Autodesk Inventor part; units mm, degrees
ref_plane "YZ Plane" through (0, 0, 0) normal (1, 0, 0) x (0, 1, 0)
ref_plane "XZ Plane" through (0, 0, 0) normal (0, 1, 0) x (-1, 0, 0)
ref_plane "XY Plane" through (0, 0, 0) normal (0, 0, 1) x (1, 0, 0)
sketch "Sketch9" plane through (0, 0, 0) normal (0, 1, 0) x (-1, 0, 0)
  line L0 (30, 30) -> (-30, 30)
  line L1 (-30, 30) -> (-30, -30)
  line L2 (-30, -30) -> (30, -30)
  line L3 (30, -30) -> (30, 30)
  line L4 (30, 30) -> (-30, -30) construction
  line L5 (-30, 30) -> (30, -30) construction
  line L6 (-28, 28) -> (28, 28)
  line L7 (28, 28) -> (28, -28)
  line L8 (28, -28) -> (-28, -28)
  line L9 (-28, -28) -> (-28, 28)
  point P0 (0, 0)
  dimension "d172" = 60
  dimension "d173" = 60
  dimension "d174" = 2
extrude "Extrusion3" add sketch "Sketch9" against normal blind 330
sketch "Sketch10" plane through (0, 0, 0) normal (1, 0, 0) x (0, 1, 0)
  line L0 (0, 30) -> (0, -30) construction
  line L1 (0, 30) -> (-330, 30) construction
  line L2 (-330, -30) -> (-330, 30) construction
  line L3 (0, -30) -> (-330, -30) construction
  line L4 (0, 0) -> (40, 0)
  line L5 (-85.25, -15.25) -> (-85.25, 15.25)
  line L6 (-85.25, 15.25) -> (-54.75, 15.25)
  line L7 (-54.75, 15.25) -> (-54.75, -15.25)
  line L8 (-54.75, -15.25) -> (-85.25, 15.25) construction
  line L9 (-85.25, -15.25) -> (-54.75, 15.25) construction
  circle A0 centre (-93, 23) radius 2.5
  circle A1 centre (-47, 23) radius 2.5
  line L10 (-85.25, -15.25) -> (-93, -23) construction
  circle A2 centre (-47, -23) radius 2.5
  circle A3 centre (-93, -23) radius 2.5
  circle A4 centre (-70, 0) radius 32.5269 construction
  line L11 (-54.75, -15.25) -> (-85.25, -15.25)
  line L12 (-44.5, -25.5) -> (-95.5, -25.5) construction
  line L13 (-95.5, -25.5) -> (-95.5, 25.5) construction
  line L14 (-95.5, 25.5) -> (-44.5, 25.5) construction
  line L15 (-44.5, 25.5) -> (-44.5, -25.5) construction
  line L16 (-44.5, -25.5) -> (-95.5, 25.5) construction
  line L17 (-95.5, -25.5) -> (-44.5, 25.5) construction
  line L18 (-70, 37.0891) -> (-70, 0) construction
  circle A5 centre (-93, 23) radius 10.9602 construction
  point P0 (-391.3995, 90.0207)
  point P1 (-386.6495, 165.0207)
  dimension "d191" = 21.9203
  dimension "d181" = 40
  dimension "d187" = 30.5
  dimension "d188" = 30.5
  dimension "d189" = 5
  dimension "d190" = 51
  dimension "d192" = 110
  dimension "d196" = 46
extrude "Extrusion4" cut sketch "Sketch10" along normal through all both and the other way through all
pattern_linear "Rectangular Pattern4" count 3 spacing 110 along (0, -1, 0) of "Extrusion4"
properties part number "PRS 1200-55 (fds) main way tube" material "Stainless Steel"
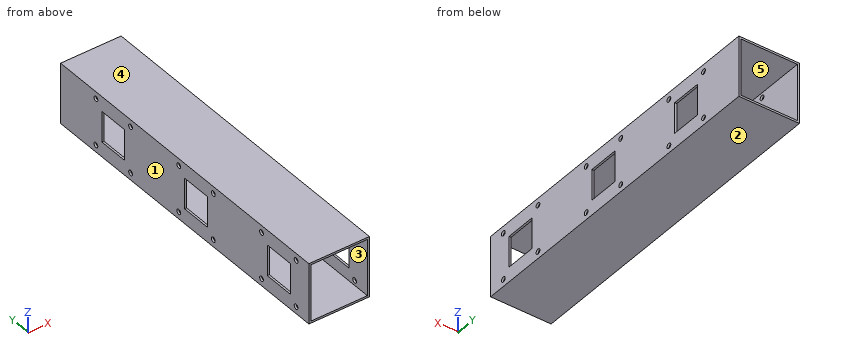
Check sheet for the modelled part. Datum: model origin and axes. Units: mm. Face numbers are marked on the shaded views. A direction names the side the tool comes from. Coordinates: 2 decimals unless noted, no trailing zeros. Write each loop counter-clockwise with the first axis right and the second up, starting at its lowest first coordinate (ties: lowest second). Pieces come first, ordered by that corner, then holes. Notation, with made-up numbers: M -6.75,26 L 2.25,26 A36 ccw 2.25,65 Z; hole C 47.5,-24.5 d7. An arc over 180 degrees is marked long. Use one line per item in the form item = value.
Item 1: Sectioned sample at D-D, the plane y = -103. Record the cut outline in (x, z).
Answer below:
outline = M -30,-30 L 30,-30 L 30,30 L -30,30 Z; hole M -28,-28 L 28,-28 L 28,28 L -28,28 Z
Item 2: Gauge pin test, flat end, axial feed: pin 1 Ø4.5 at (y, z) = (-93, 23) entering from -X (3 decimals). Record the tip position at first contact, or that the pin passes through.
Answer below:
pin_1 = through
Item 3: Sectioned sample at C-C, the plane y = -186.5. Record the cut outline in (x, z).
Answer below:
outline = M -30,-30 L 30,-30 L 30,-15.25 L 28,-15.25 L 28,-28 L -28,-28 L -28,-15.25 L -30,-15.25 Z; M -30,15.25 L -28,15.25 L -28,28 L 28,28 L 28,15.25 L 30,15.25 L 30,30 L -30,30 Z
Item 4: Material ranges on L1, parallel to Z at x = -28.8, y = -93; L2, parallel to Z at x = -24.5, y = -259, recorded low to high. Write a range as from..to.
Answer below:
L1 = -30..-25.5, -20.5..20.5, 25.5..30
L2 = -30..-28, 28..30
Item 5: Sectioned sample at B-B, the plane x = 18.5. Record the cut outline in (y, z).
Answer below:
outline = M -330,-30 L 0,-30 L 0,-28 L -330,-28 Z; M -330,28 L 0,28 L 0,30 L -330,30 Z
Item 6: Sectioned sample at A-A, the plane z = -4.5. State how many separate pieces and enclosed holes the cut face has, and give its area (3 significant figures).
Answer below:
separate_pieces = 8
enclosed_holes = 0
area = 954 mm^2
Item 7: Release check for a two-part mould opening along Z. For the marked faces 1, 2 and 3 record: pulls with the +Z half, pulls with the -Z half, needs draft (parallel to the pull), parting line crosses it, or undercut.
Answer below:
face_1 = needs draft
face_2 = pulls with the -Z half
face_3 = undercut
Item 8: Set-up check for the marked faces 4 and 5: record each of +Z, -Z, +X, -X, +Y, -Y from which the full face is reachable in a straight line by a thin tool's end or side.
Answer below:
face_4 = +Z, +X, -X, +Y, -Y
face_5 = +Y, -Y
